The model under review builds one solid part; all positions refer to its coordinate system, in mm. A direction names the side the tool comes from. Round coordinates to 2 decimals unless told otherwise and drop trailing zeros. Loops run counter-clockwise (first coordinate to the right, second up) from the corner with the lowest first, then second, coordinate; pieces in that order, holes last. Notation, with made-up numbers: M 26,-2.5 L 33,-2.5 A11 ccw 33,14.5 Z; hole C 9.5,-2 d5. An arc over 180 degrees is marked long. Use a Markdown table: item, result. Add a question column.
```python
from build123d import *

# Parameters (mm, degrees)
SKETCH1_W           = 34
SKETCH1_H           = 28
BOSS_EXTRUDE1_DEPTH = 9
CUT_EXTRUDE1_DEPTH  = 8.5
CUT_EXTRUDE2_DEPTH  = 9
CUT_EXTRUDE3_DEPTH  = 9
SKETCH6_W           = 2.295965215
SKETCH6_H           = 4.061171394
CUT_EXTRUDE4_DEPTH  = 9
SKETCH7_W           = 3.765813474
SKETCH7_H           = 2.196724527
CUT_EXTRUDE5_DEPTH  = 9


with BuildPart() as part:
    # Sketch1 → Boss-Extrude1 (new body)
    with BuildSketch(Plane(origin=(0, 0, 0), x_dir=(1, 0, 0), z_dir=(0, 1, 0))):
        with Locations((1.757158316, -7.233665399)):
            Rectangle(SKETCH1_W, SKETCH1_H)
    extrude(amount=BOSS_EXTRUDE1_DEPTH)

    # Sketch3 → Cut-Extrude1 (cut)
    with BuildSketch(Plane(origin=(0, 9, 0), x_dir=(1, 0, 0), z_dir=(0, 1, 0))):
        Polygon((-13.709642768, 6.266334601), (-14.742841684, 4.916334601), (-14.742841684, -17.206480141), (-14.742841684, -20.733665399), (18.257158316, -20.733665399), (18.257158316, 5.046334601), (16.903908894, 6.266334601), align=None)
    extrude(amount=-CUT_EXTRUDE1_DEPTH, mode=Mode.SUBTRACT)

    # Sketch4 → Cut-Extrude2 (cut)
    with BuildSketch(Plane(origin=(0, 9, 0), x_dir=(1, 0, 0), z_dir=(0, 1, 0))):
        with BuildLine():
            Line((-15.242841684, 5.703653574), (-15.242841684, 6.766334601))
            Line((-15.242841684, 6.766334601), (-14.184858911, 6.765079364))
            ThreePointArc((-14.184858911, 6.765079364), (-14.926543667, 6.446369911), (-15.242841684, 5.703653574))
        make_face()
        with BuildLine():
            Line((18.763393814, 5.6549421), (18.757158316, 6.766334601))
            Line((18.757158316, 6.766334601), (17.66754215, 6.766334601))
            ThreePointArc((17.66754215, 6.766334601), (18.434091592, 6.4262049), (18.763393814, 5.6549421))
        make_face()
    extrude(amount=-CUT_EXTRUDE2_DEPTH, mode=Mode.SUBTRACT)

    # Sketch5 → Cut-Extrude3 (cut)
    with BuildSketch(Plane(origin=(0, 9, 0), x_dir=(1, 0, 0), z_dir=(0, 1, 0))):
        Polygon((-14.184858911, 6.765079364), (-14.181243432, 6.766334601), (-15.374291847, 6.820902747), (-15.330265958, 6.661105077), align=None)
    extrude(amount=-CUT_EXTRUDE3_DEPTH, mode=Mode.SUBTRACT)

    # Sketch6 → Cut-Extrude4 (cut)
    with BuildSketch(Plane(origin=(0, 0.5, 0), x_dir=(1, 0, 0), z_dir=(0, 1, 0))):
        with Locations((2.314867695, -4.634515707)):
            Rectangle(SKETCH6_W, SKETCH6_H)
    extrude(amount=-CUT_EXTRUDE4_DEPTH, mode=Mode.SUBTRACT)

    # Sketch7 → Cut-Extrude5 (cut)
    with BuildSketch(Plane(origin=(18.757158316, 0, 0), x_dir=(0, 0, -1), z_dir=(1, 0, 0))):
        with Locations((-5.821485346, 5.253162695)):
            Rectangle(SKETCH7_W, SKETCH7_H)
    extrude(amount=-CUT_EXTRUDE5_DEPTH, mode=Mode.SUBTRACT)


solid = part.part
```
(1) For faces 4 (the face through (2, 5, 20.734)), 5 (the face through (18.757, 4, 8)), list the 3-axis set-ups (+Z, -Z, +X, -X, +Y, -Y) from which the entire face can be reached by the end or side of a thin tool; tool diameter is ignored.
(2) Draft analysis for pull direction Z (two halves, no side actions). For faces 1 (the face through (2, 4, -6.766)), 2 (the face through (2, 0.5, 7)), 3 (the face through (-15.243, 4, 8)), state which applies: released by +Z, released by -Z, zero draft, split by the parting line, or undercut.
(3) Insertion check: pin 1 Ø8 at (x, z) = (5.5, 11.5) entering from +Y; pin 2 Ø0.6 at (x, y) = (18.5, 5.5) entering from -Z. Each pin has a flat end and moves straight along its axis. Give the tip position at first contact, or say it passes through.
(4) To check wall thickness, follow probe 1 along Z at (x, y) = (-0.5, 0.75); probe 2 along X at (y, z) = (2, -0.25); probe 3 along Y at (x, z) = (10, 6.5). State the ranges of each line that lie inside material, in increasing order.
(5) Consider section A-A, the plane x = 3. Give the boundary of the cut face in (y, z).
(6) Consider section C-C, the plane z = 12.75. Give the boundary of the cut face in (x, y), then the cut area to 3 significant figures.
Found:
| question | item | result |
|---|---|---|
| 1 | face 4 | +Y |
| 1 | face 5 | +Z, -Z, +X, +Y, -Y |
| 2 | face 1 | released by -Z |
| 2 | face 2 | undercut |
| 2 | face 3 | zero draft |
| 3 | pin 1 | stops at y = 0.5 |
| 3 | pin 2 | stops at z = -6.61 |
| 4 | probe 1 | z = -6.77 to -6.27, 20.73 to 21.23 |
| 4 | probe 2 | x = -15.24 to -14.74, 18.26 to 18.76 |
| 4 | probe 3 | y = 0 to 0.5 |
| 5 | outline | M 0,-6.77 L 9,-6.77 L 9,-6.27 L 0.5,-6.27 L 0.5,2.6 L 0,2.6 Z; M 0,6.67 L 0.5,6.67 L 0.5,20.73 L 9,20.73 L 9,21.23 L 0,21.23 Z |
| 6 | outline | M -15.24,0 L 18.76,0 L 18.76,9 L 18.26,9 L 18.26,0.5 L -14.74,0.5 L -14.74,9 L -15.24,9 Z |
| 6 | area | 25.5 mm^2 |
